from build123d import *

# Parameters (mm, degrees)
F0_W     = 266.7
F0_H     = 152.4
F0_R     = 19.05
F1_DEPTH = 50.8
F2_R     = 6.35


with BuildPart() as f1:
    # F0 (on Top) → F1 (new body)
    with BuildSketch(Plane.XY):
        Rectangle(F0_W, F0_H)
        with BuildLine():
            ThreePointArc((82.549939, -0.048241), (63.475818, -19.098226), (44.45, 0))
            ThreePointArc((44.45, 0), (63.52406, 19.001743), (82.549939, -0.048241))
        make_face(mode=Mode.SUBTRACT)
        with Locations((-63.5, 0)):
            Circle(F0_R, mode=Mode.SUBTRACT)
        with BuildLine():
            ThreePointArc((-19.05, 0), (0, 19.05), (19.05, 0))
            ThreePointArc((19.05, 0), (0, -19.05), (-19.05, 0))
        make_face(mode=Mode.SUBTRACT)
    extrude(amount=F1_DEPTH)

    # F2
    f2_edges = [f1.edges().sort_by_distance(p)[0] for p in [
        (0, -76.2, 50.8),
        (133.35, 0, 50.8),
        (0, 76.2, 50.8),
        (-133.35, 0, 50.8),
    ]]
    fillet(f2_edges, radius=F2_R)


solid = f1.part
Can you work these out from the model? Positions are in its coordinate system, mm. Round coordinates to 2 decimals unless told otherwise and drop trailing zeros. Loops run counter-clockwise (first coordinate to the right, second up) from the corner with the lowest first, then second, coordinate; pieces in that order, holes last. Notation, with made-up numbers: (9.5, 61) - (30.5, 61) arc R28 cw to (30.5, 95) - close; hole circle Ø9 at (-10, -20.5). An arc over 180 degrees is marked (long way). Use CSV: the item, a comma, the result in double quotes. Start each with the question number.
1) If we section it at B-B on z = 8.5: Write out the boundary of the cut face in (x, y), plus the area to 3 significant figures.
2) For pin 1 Ø12 at (x, y) = (93, -31) entering from -Z, with a flat end and sliding along its axis, tell me the tip position at first contact or that it passes through.
3) If we section it at D-D on x = 0.5: Write out the boundary of the cut face in (y, z), plus the area to 3 significant figures.
4) If we section it at A-A on x = -63.5: Write out the boundary of the cut face in (y, z), plus the area to 3 significant figures.
5) If we section it at C-C on y = 3: Write out the boundary of the cut face in (x, z).
6) We'd pull the mould along X, two halves only. Please class faces 1 (the flat face through (26, 1, 50.8)), 2 (the cylindrical face through (-15.12, 11.59, 25.04)), 3 (the flat face through (-133.35, -1, 22)): released by +X, released by -X, zero draft, split by the parting line, or undercut.
7) Please list where these lines run through material, in increasing order: probe 1 along Y at (x, z) = (-63, 29); probe 2 along X at (y, z) = (-3.5, 19); probe 3 along Y at (x, z) = (3, 8). Write a range as [from, to].
Geometry results:
1,outline,"(-133.35, -76.2) - (133.35, -76.2) - (133.35, 76.2) - (-133.35, 76.2) - close; hole circle Ø38.1 at (-63.5, 0); hole circle Ø38.1 at (0, 0); hole circle Ø38.1 at (63.5, -0.05)"
1,area,"37,200 mm2"
2,pin 1,"stops at z = 0"
3,outline,"(-76.2, 0) - (-19.04, 0) - (-19.04, 50.8) - (-69.85, 50.8) arc R6.35 ccw to (-76.2, 44.45) - close; (19.04, 0) - (76.2, 0) - (76.2, 44.45) arc R6.35 ccw to (69.85, 50.8) - (19.04, 50.8) - close"
3,area,"5,790 mm2"
4,outline,"(-76.2, 0) - (-19.05, 0) - (-19.05, 50.8) - (-69.85, 50.8) arc R6.35 ccw to (-76.2, 44.45) - close; (19.05, 0) - (76.2, 0) - (76.2, 44.45) arc R6.35 ccw to (69.85, 50.8) - (19.05, 50.8) - close"
4,area,"5,790 mm2"
5,outline,"(-133.35, 0) - (-82.31, 0) - (-82.31, 50.8) - (-127, 50.8) arc R6.35 ccw to (-133.35, 44.45) - close; (-44.69, 0) - (-18.81, 0) - (-18.81, 50.8) - (-44.69, 50.8) - close; (18.81, 0) - (44.7, 0) - (44.7, 50.8) - (18.81, 50.8) - close; (82.3, 0) - (133.35, 0) - (133.35, 44.45) arc R6.35 ccw to (127, 50.8) - (82.3, 50.8) - close"
6,face 1,"zero draft"
6,face 2,"undercut"
6,face 3,"released by -X"
7,probe 1,"y = [-76.2, -19.04], [19.04, 76.2]"
7,probe 2,"x = [-133.35, -82.23], [-44.77, -18.73], [18.73, 44.77], [82.23, 133.35]"
7,probe 3,"y = [-76.2, -18.81], [18.81, 76.2]"
